```python
from build123d import *

# Parameters (mm, degrees)
BOSS_EXTRUDE1_DEPTH = 300


with BuildPart() as part:
    # Sketch1 → Boss-Extrude1 (new body)
    with BuildSketch(Plane.XY):
        with BuildLine():
            Line((0, -5), (0, -10))
            Line((0, -10), (-3, -10))
            Line((-3, -10), (-3, 0.518235133))
            Line((-3, 0.518235133), (-8.952395517, -1.422763405))
            Line((-8.952395517, -1.422763405), (1.422311977, -33.238533054))
            ThreePointArc((1.422311977, -33.238533054), (12.993401498, -40.316712963), (21.8, -30))
            Line((21.8, -30), (21.8, -10))
            Line((21.8, -10), (21.3, -10))
            Line((21.3, -10), (21.3, -5))
            Line((21.3, -5), (0, -5))
        make_face()
    extrude(amount=-BOSS_EXTRUDE1_DEPTH)


solid = part.part
```
Geometry check sheet. Reference: the model listing, model coordinates, mm. A direction names the side the tool comes from. Round coordinates to 2 decimals unless told otherwise and drop trailing zeros. Loops run counter-clockwise (first coordinate to the right, second up) from the corner with the lowest first, then second, coordinate; pieces in that order, holes last. Notation, with made-up numbers: M 16,2 L 74,2 A4 ccw 74,9 Z; hole C -33,-35.5 d1. An arc over 180 degrees is marked long. Return JSON: item names as keys, results as strings. Group by question number.
(1) Go/stop test with flat-tipped pins: pin 1 (5.5 mm diameter, centred on y = -7.5, z = -170.5, fed in from +X); pin 2 (17 mm diameter, centred on x = 13.5, z = -134, fed in from +Y); pin 3 (5.5 mm diameter, centred on y = -3, z = -163, fed in from +X); pin 4 (1.5 mm diameter, centred on x = -1.5, z = -215.5, fed in from +Y). Record where each tip stops, or that it passes through.
(2) Section check A-A, the plane z = -235. Enter the section's corners in (x, y).
(3) Section check C-C, the plane y = -14. Enter the section's corners in (x, z), and give its area (3 significant figures).
(4) Mould release check, pull along X, two halves, no side actions. Record for faces 3 (the face through (0, -7, -148)), 4 (the face through (21.8, -20, -148)), 5 (the face through (11, -5, -148)), 6 (the face through (-3, -5, -148)): pulls with the +X half, pulls with the -X half, needs draft (parallel to the pull), parting line crosses it, or undercut.
(5) Scan lines: line 1 along X through (y, z) = (-9, -231.5); line 2 along Y through (x, z) = (12, -23); line 3 along X through (y, z) = (-36.5, -62). Record each from-to range of solid material in increasing order. Write a range as [from, to].
(6) Section check B-B, the plane x = 17. Enter the section's corners in (y, z).
(7) Set-up check for faces 1 (the face through (21.3, -8, -148)), 2 (the face through (10, -20, 0)): record each of +Z, -Z, +X, -X, +Y, -Y from which the full face is reachable in a straight line by a thin tool's end or side.
Data:
{
 "1": {"pin 1": "x = 21.8", "pin 2": "y = -5", "pin 3": "x = 21.3", "pin 4": "y = -10"},
 "2": {"outline": "M -8.95,-1.42 L 1.42,-33.24 A10.45 ccw 21.8,-30 L 21.8,-10 L 21.3,-10 L 21.3,-5 L 0,-5 L 0,-10 L -3,-10 L -3,0.52 Z"},
 "3": {"outline": "M -4.85,-300 L 21.8,-300 L 21.8,0 L -4.85,0 Z", "area": "8,000 mm²"},
 "4": {"face 3": "undercut", "face 4": "pulls with the +X half", "face 5": "needs draft", "face 6": "undercut"},
 "5": {"line 1": "[-6.48, -3], [0, 21.3]", "line 2": "[-40.43, -5]", "line 3": "[3.18, 19.53]"},
 "6": {"outline": "M -38.79,-300 L -5,-300 L -5,0 L -38.79,0 Z"},
 "7": {"face 1": "+Z, -Z, +X, +Y", "face 2": "+Z, +X, -X, +Y, -Y"}
}
